The model under review builds one solid part; all positions refer to its coordinate system, in mm. Coordinates: 2 decimals unless noted, no trailing zeros. Loops run counter-clockwise (first coordinate to the right, second up) from the corner with the lowest first, then second, coordinate; pieces in that order, holes last. Notation, with made-up numbers: (52, 50.25) - (63, 50.25) arc R15 ccw to (63, 71.25) - close; hole circle Ø11 at (75.5, -32.5). An arc over 180 degrees is marked (long way). Use a Markdown table: item, result. Add a question column.
1) Add section B-B, the plane z = 0. Give the boundary of the cut face in (x, y) (3 decimals), and give its area (3 significant figures).
2) The part is to be moulded in two halves that separate along Z. For faces 1 (the flat face through (-1, 9, 85.725)), 2 (the cylindrical face through (64.09, 9.26, 63.62)), 3 (the flat face through (-1, 0, -20)), say which applies: pulls with the +Z half, pulls with the -Z half, needs draft (parallel to the pull), parting line crosses it, or undercut.
3) Add section A-A, the plane x = 0. Give the boundary of the cut face in (y, z) (3 decimals), and give its area (3 significant figures).
4) To check wall thickness, follow L1, parallel to Z at x = 0, y = 7 (3 decimals); L2, parallel to Z at x = -61, y = 9 (3 decimals); L3, parallel to X at y = 9.5, z = -64. State the ranges of each line that lie inside material, in increasing order. Write a range as [from, to].
```python
from build123d import *

# Parameters (mm, degrees)
SKETCH1_W                  = 171.45
SKETCH1_H                  = 171.45
BOSS_EXTRUDE1_DEPTH        = 18.25625
SKETCH2_R                  = 17.4625
CUT_EXTRUDE1_DEPTH         = 123.60033407
F_1_2_0_5_DIAMETER_HOLE1_D = 12.7


with BuildPart() as part:
    # Sketch1 → Boss-Extrude1 (new body)
    with BuildSketch(Plane(origin=(0, 0, 0), x_dir=(1, 0, 0), z_dir=(0, 1, 0))):
        Rectangle(SKETCH1_W, SKETCH1_H)
    extrude(amount=BOSS_EXTRUDE1_DEPTH)

    # Sketch2 → Cut-Extrude1 (cut, through all)
    with BuildSketch(Plane(origin=(0, 18.25625, 0), x_dir=(1, 0, 0), z_dir=(0, 1, 0))):
        with Locations((-76.2, 76.2)):
            Circle(SKETCH2_R)
        with Locations((76.2, 76.2)):
            Circle(SKETCH2_R)
        with Locations((76.2, -76.2)):
            Circle(SKETCH2_R)
        with Locations((-76.2, -76.2)):
            Circle(SKETCH2_R)
    extrude(amount=-CUT_EXTRUDE1_DEPTH, mode=Mode.SUBTRACT)

    # 1/2 (0.5) Diameter Hole1 (through all)
    with Locations(Plane(origin=(0, 18.25625, 0), x_dir=(1, 0, 0), z_dir=(0, 1, 0))):
        with Locations((0, 0)):
            Hole(F_1_2_0_5_DIAMETER_HOLE1_D / 2)


solid = part.part
```
From the geometry:
| question | item | result |
|---|---|---|
| 1 | outline | (-85.725, 0) - (-6.35, 0) - (-6.35, 18.256) - (-85.725, 18.256) - close; (6.35, 0) - (85.725, 0) - (85.725, 18.256) - (6.35, 18.256) - close |
| 1 | area | 2,900 mm^2 |
| 2 | face 1 | pulls with the +Z half |
| 2 | face 2 | undercut |
| 2 | face 3 | needs draft |
| 3 | outline | (0, -85.725) - (18.256, -85.725) - (18.256, -6.35) - (0, -6.35) - close; (0, 6.35) - (18.256, 6.35) - (18.256, 85.725) - (0, 85.725) - close |
| 3 | area | 2,900 mm^2 |
| 4 | L1 | z = [-85.725, -6.35], [6.35, 85.725] |
| 4 | L2 | z = [-85.725, -84.796], [-67.604, 67.604], [84.796, 85.725] |
| 4 | L3 | x = [-63.71, 63.71] |
